Check sheet for the modelled part. Datum: model origin and axes. Units: mm. Coordinates: 2 decimals unless noted, no trailing zeros. Write each loop counter-clockwise with the first axis right and the second up, starting at its lowest first coordinate (ties: lowest second). Pieces come first, ordered by that corner, then holes. Notation, with made-up numbers: (45, 63) -> (59, 63) arc R26 ccw to (59, 80) -> close; hole circle Ø5 at (-12, 41). An arc over 180 degrees is marked (long way). One line per item, written item: value. Start each with the question number.
1) Sectioned sample at C-C on y = 33.4. Enter the section's corners in (x, z).
2) Sectioned sample at A-A on z = 0.5. Enter the section's corners in (x, y).
3) Sectioned sample at B-B on x = 18.4. Enter the section's corners in (y, z), plus the area to 3 significant figures.
4) Draft check along Y on faces 1 (the cylindrical face through (53.3, 1.43, 1.01)), 2 (the cylindrical face through (19.74, 35.51, 0.99)), 3 (the flat face through (27, 40, 0)). Enter one of: +Y half, -Y half, draft (parallel to the pull), parting line (faces both ways), or undercut.
5) Scan lines: line 1 along Y through (x, z) = (18.4, 1.5); line 2 along Y through (x, z) = (16.5, 0.6); line 3 along X through (y, z) = (23, 0.8). Record each from-to range of solid material in increasing order. Write a range as [from, to].
```python
from build123d import *

# Parameters (mm, degrees)
F0_W     = 54.8
F0_H     = 79.2
F0_R     = 2.5
F1_DEPTH = 2
F2_R     = 5


with BuildPart() as f1:
    # F0 (on Top) → F1 (new body)
    with BuildSketch(Plane.XY):
        with Locations((27.4, 39.6)):
            Rectangle(F0_W, F0_H)
        with Locations((18.4, 21.4)):
            Circle(F0_R, mode=Mode.SUBTRACT)
        with Locations((18.4, 33.4)):
            Circle(F0_R, mode=Mode.SUBTRACT)
        with Locations((36.4, 21.4)):
            Circle(F0_R, mode=Mode.SUBTRACT)
        with Locations((36.4, 33.4)):
            Circle(F0_R, mode=Mode.SUBTRACT)
    extrude(amount=F1_DEPTH)

    # F2
    f2_edges = [f1.edges().sort_by_distance(p)[0] for p in [
        (54.8, 0, 1),
        (0, 0, 1),
    ]]
    fillet(f2_edges, radius=F2_R)


solid = f1.part
```
Answers:
1. outline: (0, 0) -> (15.9, 0) -> (15.9, 2) -> (0, 2) -> close; (20.9, 0) -> (33.9, 0) -> (33.9, 2) -> (20.9, 2) -> close; (38.9, 0) -> (54.8, 0) -> (54.8, 2) -> (38.9, 2) -> close
2. outline: (0, 5) arc R5 ccw to (5, 0) -> (49.8, 0) arc R5 ccw to (54.8, 5) -> (54.8, 79.2) -> (0, 79.2) -> close; hole circle Ø5 at (18.4, 21.4); hole circle Ø5 at (18.4, 33.4); hole circle Ø5 at (36.4, 21.4); hole circle Ø5 at (36.4, 33.4)
3. outline: (0, 0) -> (18.9, 0) -> (18.9, 2) -> (0, 2) -> close; (23.9, 0) -> (30.9, 0) -> (30.9, 2) -> (23.9, 2) -> close; (35.9, 0) -> (79.2, 0) -> (79.2, 2) -> (35.9, 2) -> close
3. area: 138 mm2
4. face 1: -Y half
4. face 2: undercut
4. face 3: draft
5. line 1: y = [0, 18.9], [23.9, 30.9], [35.9, 79.2]
5. line 2: y = [0, 19.78], [23.02, 31.78], [35.02, 79.2]
5. line 3: x = [0, 16.48], [20.32, 34.48], [38.32, 54.8]
